CAD build for the part. Positions are in the model's coordinates, mm. Face numbers are marked on the shaded views. A direction names the side the tool comes from. Give positions to 0.01 mm unless a question says otherwise; leave off trailing zeros. Write each loop counter-clockwise with the first axis right and the second up, starting at its lowest first coordinate (ties: lowest second). Pieces come first, ordered by that corner, then holes. Notation, with made-up numbers: (-17, 58.25) - (13, 58.25) arc R10 ccw to (13, 62.25) - close; hole circle Ø9 at (48.25, 44.25). An arc over 180 degrees is marked (long way). Answer as a JSON object with one key per item and string values.
Autodesk Inventor part; units mm, degrees
ref_plane "YZ Plane" through (0, 0, 0) normal (1, 0, 0) x (0, 1, 0)
ref_plane "XZ Plane" through (0, 0, 0) normal (0, 1, 0) x (-1, 0, 0)
ref_plane "XY Plane" through (0, 0, 0) normal (0, 0, 1) x (1, 0, 0)
sketch "Sketch1" plane through (0, 0, 0) normal (0, 1, 0) x (-1, 0, 0)
  circle A0 centre (0, 0) radius 0.825
  dimension "d0" = 1.65
extrude "Extrusion1" add sketch "Sketch1" along normal blind 0.605
sketch "Sketch2" plane through (0, 0.605, 0) normal (0, 1, 0) x (1, 0, 0)
  circle A0 centre (0, 0) radius 0.825
  circle A1 centre (0, 0) radius 0.66
  dimension "d3" = 1.32
extrude "Extrusion2" add sketch "Sketch2" along normal blind 6.96 contours A1
sketch "Sketch3" plane through (0, 7.565, 0) normal (0, 1, 0) x (1, 0, 0)
  circle A0 centre (0, 0) radius 0.715
  dimension "d6" = 1.43
extrude "Extrusion3" add sketch "Sketch3" along normal blind 0.6875
chamfer "Chamfer1" distance 0.055 angle 45 2 edges at (-0.715, 8.2525, 0) (-0.715, 7.565, 0)
sketch "Sketch4" plane through (0, 0, 0) normal (0, 0, 1) x (1, 0, 0)
  line L0 (-0.66, 8.2525) -> (0.66, 8.2525)
  line L1 (0, 8.2525) -> (0.0412, 8.2525)
  line L2 (0.0412, 8.2525) -> (0.0412, 5.5025)
  line L3 (0.0412, 5.5025) -> (0, 5.5025)
  circle A0 centre (0, 5.5025) radius 0.0412
  line L4 (0, 5.5025) -> (0, 5.524)
  line L5 (-0.0412, 8.2525) -> (-0.0412, 5.5025)
  line L6 (-0.0412, 8.2525) -> (0, 8.2525)
  point P0 (0, 0)
  dimension "d12" = 0.0413
  dimension "d13" = 2.75
extrude "Extrusion4" cut sketch "Sketch4" against normal mid plane 2.1875
pattern_circular "Circular Pattern1" count 4 over 360 about axis through (0, 0.605, 0) along (0, 1, 0) of "Extrusion4"
properties part number "Pin_Dedao"
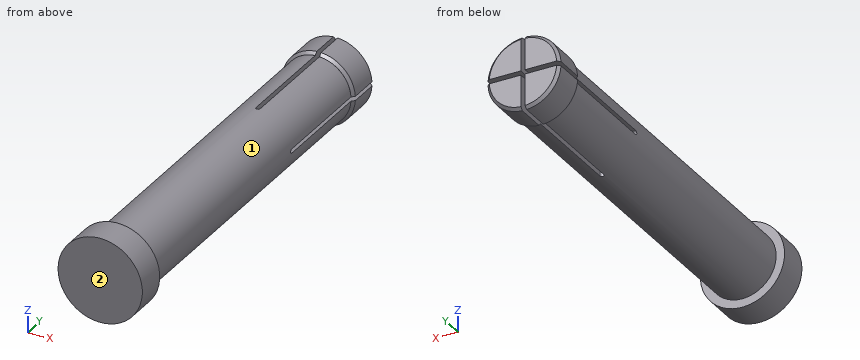
(1) 3-axis set-ups, long thin cutter, end or side, ignore diameter. For the marked faces 1 and 2: which of +Z, -Z, +X, -X, +Y, -Y reach the whole face in a straight line?
Answer key:
{"face 1": "none", "face 2": "+Z, -Z, +X, -X, -Y"}
(2) Saw through at A-A, the plane y = 6.5. Give the cut face in (x, z), and give its area (3 significant figures).
Answer key:
{"outline": "(-0.66, -0.04) arc R0.66 ccw to (-0.04, -0.66) - (-0.04, -0.04) - close; (-0.66, 0.04) - (-0.04, 0.04) - (-0.04, 0.66) arc R0.66 ccw to start; (0.04, -0.66) arc R0.66 ccw to (0.66, -0.04) - (0.04, -0.04) - close; (0.04, 0.04) - (0.66, 0.04) arc R0.66 ccw to (0.04, 0.66) - close", "area": "1.16 mm²"}
(3) Saw through at B-B, the plane y = 2.25. Give the cut face in (x, z).
Answer key:
{"outline": "circle Ø1.32 at (0, 0)"}
(4) Flat gauge pins, fed straight in: P1, Ø0.5, axis at x = -0.5, y = 7.5, coming from the +Z side; P2, Ø0.5, axis at y = 7, z = -0.5, coming from the -X side; P3, Ø0.7, axis at y = 7.5, z = -0.5, coming from the +X side. Where does each tip first touch, or does it go through?
Answer key:
{"P1": "stops at z = 0.66", "P2": "stops at x = -0.61", "P3": "stops at x = 0.69"}
(5) Probe L1, parallel to Z at x = 0.05, y = 3.25; L2, parallel to Y at x = -0.55, z = -0.5 (3 decimals); L3, parallel to Z at x = 0.3, y = 5.25. List the from-to ranges inside material, lowest first. Write a range as [from, to].
Answer key:
{"L1": "z = [-0.66, 0.66]", "L2": "y = [0, 0.605]", "L3": "z = [-0.59, 0.59]"}
